Solid Edge part; units mm, degrees
sketch "Sketch1" plane through (0, 0, 0) normal (0, -1, 0) x (1, 0, 0)
  line L0 (-24.5, -16.25) -> (24.5, -16.25)
  line L1 (24.5, -16.25) -> (24.5, 16.25)
  line L2 (24.5, 16.25) -> (-24.5, 16.25)
  line L3 (-24.5, 16.25) -> (-24.5, -16.25)
extrude "Protrusion1" add sketch "Sketch1" against normal blind 3
sketch "Sketch2" plane through (0, 0, 0) normal (0, -1, 0) x (1, 0, 0)
  line L0 (-19.5, -3.75) -> (19.5, -3.75)
  line L1 (19.5, -3.75) -> (19.5, -16.25)
  line L2 (19.5, -16.25) -> (-19.5, -16.25)
  line L3 (-19.5, -16.25) -> (-19.5, -3.75)
  dimension "D1" = 19.5
  dimension "D2" = 19.5
extrude "ExtrudedCutout_1" cut sketch "Sketch2" along normal mid plane 68.2044
sketch "Sketch3" plane through (0, 0, 0) normal (0, -1, 0) x (1, 0, 0)
  circle A0 centre (-22, -13.75) radius 1.55
  circle A1 centre (22, -13.75) radius 1.55
  dimension "D1" = 22
extrude "ExtrudedCutout_2" cut sketch "Sketch3" along normal mid plane 83.9594
The model under review builds one solid part; all positions refer to its coordinate system, in mm. A direction names the side the tool comes from. Give positions to 0.01 mm unless a question says otherwise; leave off trailing zeros. Write each loop counter-clockwise with the first axis right and the second up, starting at its lowest first coordinate (ties: lowest second). Pieces come first, ordered by that corner, then holes.
1. Add section A-A, the plane z = -10.5. Write out the cut boundary in (x, y).
2. Add section D-D, the plane z = -13.75. Write out the cut boundary in (x, y), plus the area to 3 significant figures.
3. Draft analysis for pull direction Z (two halves, no side actions). For faces 1 (the flat face through (0, 2, -3.75)), 2 (the cylindrical face through (22.83, 1.48, -12.44)), 3 (the flat face through (0, 0, 4)), 4 (the cylindrical face through (-21.17, 1.48, -12.44)), state which applies: +Z half, -Z half, draft (parallel to the pull), parting line (faces both ways), or undercut.
4. For P1, Ø3, axis at x = 22, z = -13.75, coming from the -Y side, flat-tipped, find the tip position at first contact; note if it passes through.
5. Tool access review of faces 5 (the flat face through (22, 1, -16.25)), 6 (the flat face through (19.5, 2, -10)): name each direction out of +Z, -Z, +X, -X, +Y, -Y from which nothing blocks a thin tool from reaching the whole face with its end or side.
6. Wall thickness on L1, parallel to X at y = 2.5, z = -4; L2, parallel to Z at x = -22, y = 0.85; L3, parallel to Z at x = 9, y = 0.6: over which ranges is each line inside the solid? List them lowest first.
7. Add section B-B, the plane x = 22. Write out the cut boundary in (y, z), plus the area to 3 significant figures.
8. Add section C-C, the plane y = 0.7. Write out the cut boundary in (x, z), plus the area to 3 significant figures.
Worked answers:
1. outline: (-24.5, 0) - (-19.5, 0) - (-19.5, 3) - (-24.5, 3) - close; (19.5, 0) - (24.5, 0) - (24.5, 3) - (19.5, 3) - close
2. outline: (-24.5, 0) - (-23.55, 0) - (-23.55, 3) - (-24.5, 3) - close; (-20.45, 0) - (-19.5, 0) - (-19.5, 3) - (-20.45, 3) - close; (19.5, 0) - (20.45, 0) - (20.45, 3) - (19.5, 3) - close; (23.55, 0) - (24.5, 0) - (24.5, 3) - (23.55, 3) - close
2. area: 11.4 mm2
3. face 1: -Z half
3. face 2: undercut
3. face 3: draft
3. face 4: undercut
4. P1: passes through
5. face 5: -Z, +X, -X, +Y, -Y
5. face 6: -Z, +Y, -Y
6. L1: x = -24.5 to -19.5, 19.5 to 24.5
6. L2: z = -16.25 to -15.3, -12.2 to 16.25
6. L3: z = -3.75 to 16.25
7. outline: (0, -16.25) - (3, -16.25) - (3, -15.3) - (0, -15.3) - close; (0, -12.2) - (3, -12.2) - (3, 16.25) - (0, 16.25) - close
7. area: 88.2 mm2
8. outline: (-24.5, -16.25) - (-19.5, -16.25) - (-19.5, -3.75) - (19.5, -3.75) - (19.5, -16.25) - (24.5, -16.25) - (24.5, 16.25) - (-24.5, 16.25) - close; hole circle Ø3.1 at (-22, -13.75); hole circle Ø3.1 at (22, -13.75)
8. area: 1,090 mm2
